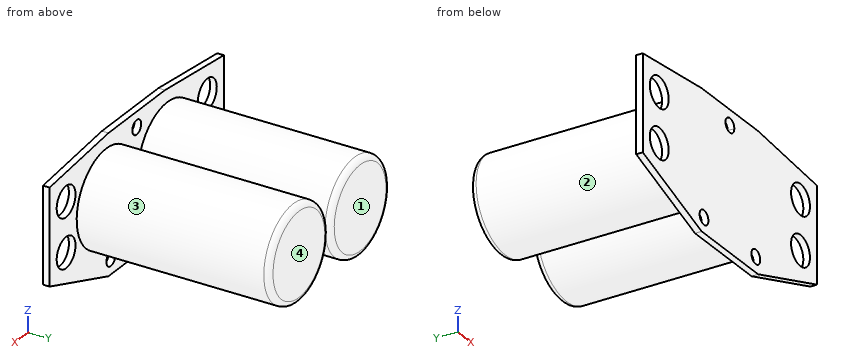
from build123d import *

# Parameters (mm, degrees)
SKETCH1_R           = 0.9525
BOSS_EXTRUDE1_DEPTH = 0.889
SKETCH3_R           = 6.35
BOSS_EXTRUDE2_DEPTH = 25.908
SKETCH2_R           = 2.032
CUT_EXTRUDE1_DEPTH  = 50.276654635
FILLET1_R           = 0.762


with BuildPart() as part:
    # Sketch1 → Boss-Extrude1 (new body)
    # profile 1 of 2: a face of its own
    with BuildSketch(Plane(origin=(0, 0, 0), x_dir=(1, 0, 0), z_dir=(0, 1, 0))):
        with BuildLine():
            Line((18.796, 2.9845), (18.796, 18.542))
            Line((18.796, 18.542), (12.7, 18.542))
            Line((12.7, 18.542), (0, 14.097))
            Line((0, 14.097), (0, 1.27))
            Line((0, 1.27), (12.7, 0))
            Line((12.7, 0), (18.796, 0))
            Line((18.796, 0), (18.796, 1.0795))
            ThreePointArc((18.796, 1.0795), (17.8435, 2.032), (18.796, 2.9845))
        make_face()
        with Locations(Location((13.208, 16.51, 0), (0, 0, 270))):
            Circle(SKETCH1_R, mode=Mode.SUBTRACT)
    # profile 2 of 2: a face of its own
    with BuildSketch(Plane(origin=(0, 0, 0), x_dir=(1, 0, 0), z_dir=(0, 1, 0))):
        with BuildLine():
            Line((24.892, 18.542), (18.796, 18.542))
            Line((18.796, 18.542), (18.796, 2.9845))
            ThreePointArc((18.796, 2.9845), (19.469519209, 2.705519209), (19.7485, 2.032))
            ThreePointArc((19.7485, 2.032), (19.469519209, 1.358480791), (18.796, 1.0795))
            Line((18.796, 1.0795), (18.796, 0))
            Line((18.796, 0), (24.892, 0))
            Line((24.892, 0), (37.592, 1.27))
            Line((37.592, 1.27), (37.592, 14.097))
            Line((37.592, 14.097), (24.892, 18.542))
        make_face()
        with Locations(Location((24.384, 16.51, 0), (0, 0, 270))):
            Circle(SKETCH1_R, mode=Mode.SUBTRACT)
    extrude(amount=BOSS_EXTRUDE1_DEPTH)

    # Sketch3 → Boss-Extrude2 (add)
    with BuildSketch(Plane(origin=(0, 0.889, 0), x_dir=(1, 0, 0), z_dir=(0, 1, 0))):
        with Locations(Location((12.192, 8.128, 0), (0, 0, 270))):
            Circle(SKETCH3_R)
        with Locations(Location((25.4, 8.128, 0), (0, 0, 270))):
            Circle(SKETCH3_R)
    extrude(amount=BOSS_EXTRUDE2_DEPTH)

    # Sketch2 → Cut-Extrude1 (cut, through all)
    with BuildSketch(Plane(origin=(0, 0.889, 0), x_dir=(1, 0, 0), z_dir=(0, 1, 0))):
        with Locations(Location((3.556, 11.303, 0), (0, 0, 270))):
            Circle(SKETCH2_R)
        with Locations(Location((3.556, 4.699, 0), (0, 0, 270))):
            Circle(SKETCH2_R)
        with Locations(Location((34.036, 4.699, 0), (0, 0, 90))):
            Circle(SKETCH2_R)
        with Locations(Location((34.036, 11.303, 0), (0, 0, 90))):
            Circle(SKETCH2_R)
    extrude(amount=-CUT_EXTRUDE1_DEPTH, mode=Mode.SUBTRACT)

    # Fillet1
    fillet1_edges = [part.edges().sort_by_distance(p)[0] for p in [
        (12.192, 26.797, -14.478),
        (25.4, 26.797, -14.478),
    ]]
    fillet(fillet1_edges, radius=FILLET1_R)


solid = part.part
The listing builds one solid part. Answer for the finished solid, in the listing's coordinates (mm). Face numbers are marked on the shaded views. A direction names the side the tool comes from. Coordinates: 2 decimals unless noted, no trailing zeros. Loops run counter-clockwise (first coordinate to the right, second up) from the corner with the lowest first, then second, coordinate; pieces in that order, holes last. Notation, with made-up numbers: M 45,12 L 87,12 A14 cw 87,18 Z; hole C 18,-6.5 d6. An arc over 180 degrees is marked long. Answer in a Markdown table with one row per item.
1) Determine the mould class of the marked faces 1 and 2 for opening direction X: released by +X, released by -X, zero draft, split by the parting line, or undercut.
Answers below:
| item | result |
|---|---|
| face 1 | zero draft |
| face 2 | undercut |
2) Find the intervals of material crossed by probe 1 along X at (y, z) = (3.25, -10.25); probe 2 along X at (y, z) = (15, -5.75); probe 3 along Z at (x, y) = (17, 19), in increasing order.
Answers below:
| item | result |
|---|---|
| probe 1 | 6.21 to 18.18, 19.42 to 31.38 |
| probe 2 | 6.3 to 18.08, 19.51 to 31.29 |
| probe 3 | -12.28 to -3.98 |
3) Which of the six approach directions +Z, -Z, +X, -X, +Y, -Y give full straight-line access (tool end or side, diameter ignored) to the marked faces 3 and 4?
Answers below:
| item | result |
|---|---|
| face 3 | +Y |
| face 4 | +Z, -Z, +X, -X, +Y |
4) Find section B-B (z = -16.51). Determine the outline of the cut face in (x, y), then the cut area to 3 significant figures.
Answers below:
| item | result |
|---|---|
| outline | M 6.89,0 L 12.26,0 L 12.26,0.89 L 6.89,0.89 Z; M 14.16,0 L 23.43,0 L 23.43,0.89 L 14.16,0.89 Z; M 25.34,0 L 30.7,0 L 30.7,0.89 L 25.34,0.89 Z |
| area | 17.8 mm^2 |
5) Find section D-D (z = -12.75). Count the separate pieces of the cut face and the enclosed holes in it, then the cut area to 3 significant figures.
Answers below:
| item | result |
|---|---|
| separate pieces | 3 |
| enclosed holes | 0 |
| area | 479 mm^2 |
6) Find section C-C (y = 20.5). Determine the outline of the cut face in (x, z), then the cut area to 3 significant figures.
Answers below:
| item | result |
|---|---|
| outline | C 12.19,-8.13 d12.7; C 25.4,-8.13 d12.7 |
| area | 253 mm^2 |
7) Find section A-A (x = 3). Determine the outline of the cut face in (y, z).
Answers below:
| item | result |
|---|---|
| outline | M 0,-15.15 L 0.89,-15.15 L 0.89,-13.26 L 0,-13.26 Z; M 0,-9.35 L 0.89,-9.35 L 0.89,-6.65 L 0,-6.65 Z; M 0,-2.74 L 0.89,-2.74 L 0.89,-0.97 L 0,-0.97 Z |
8) Given pin 1 (10 mm diameter, centred on y = 14, z = -11.5, fed in from +X); pin 2 (10 mm diameter, centred on x = 31.5, y = 8, fed in from +Z); pin 3 (4 mm diameter, centred on y = 6, z = -12.5, fed in from -X), each flat-ended and moving along its own axis, determine where each tip first touches the part or whether it passes through.
Answers below:
| item | result |
|---|---|
| pin 1 | x = 31.75 |
| pin 2 | z = -1.87 |
| pin 3 | x = 6.3 |
